```python
from build123d import *

# Parameters (mm, degrees)
F0_R     = 2.5
F1_DEPTH = 10
F2_W     = 10
F2_H     = 10
F3_DEPTH = 5
F5_DEPTH = 5


with BuildPart() as f1:
    # F0 (on Front) → F1 (new body)
    with BuildSketch(Plane.XZ):
        Circle(F0_R)
    extrude(amount=F1_DEPTH)

    # F2 (on face) → F3 (join)
    with BuildSketch(Plane.XZ.offset(10)):
        Rectangle(F2_W, F2_H)
    extrude(amount=F3_DEPTH)

    # F4 (on face) → F5 (cut, through all)
    with BuildSketch(Plane.XZ.offset(15)):
        Polygon((0, 5), (0, 0), (-5, 0), (-5, -5), (5, -5), (5, 0), (5, 5), align=None)
    extrude(amount=-F5_DEPTH, mode=Mode.SUBTRACT)


solid = f1.part
```
Verification items for the finished model (mm, model axes). A direction names the side the tool comes from. Coordinates: 2 decimals unless noted, no trailing zeros. Write each loop counter-clockwise with the first axis right and the second up, starting at its lowest first coordinate (ties: lowest second). Pieces come first, ordered by that corner, then holes. Notation, with made-up numbers: (-12, 36) - (45, 36) arc R29 ccw to (45, 58) - close; hole circle Ø11 at (88, 89). An arc over 180 degrees is marked (long way). Write item = value, one per line.
Q1. Go/stop test with flat-tipped pins: pin 1 Ø2.5 at (x, y) = (-3.5, -12) entering from -Z; pin 2 Ø1.5 at (x, y) = (-2, -8.5) entering from +Z; pin 3 Ø2.5 at (y, z) = (-12, 2.5) entering from +X. Record where each tip stops, or that it passes through.
Answer:
pin_1 = 0
pin_2 = 2.17
pin_3 = 0
Q2. Cross-section at D-D (z = 2.25). Enter the section's corners in (x, y).
Answer:
outline = (-5, -15) - (0, -15) - (0, -10) - (1.09, -10) - (1.09, 0) - (-1.09, 0) - (-1.09, -10) - (-5, -10) - close
Q3. Material ranges on L1, parallel to X at y = -14, z = 4.5; L2, parallel to Y at x = 0.75, z = -2; L3, parallel to Y at x = -3.5, z = 2, recorded low to high. Write a range as from..to.
Answer:
L1 = -5..0
L2 = -10..0
L3 = -15..-10
Q4. Cross-section at A-A (z = 0.25). Enter the section's corners in (x, y).
Answer:
outline = (-5, -15) - (0, -15) - (0, -10) - (2.49, -10) - (2.49, 0) - (-2.49, 0) - (-2.49, -10) - (-5, -10) - close
Q5. Mould release check, pull along Z, two halves, no side actions. Record for faces 1 (the face through (-5, -12, 2)), 2 (the face through (-2, -13, 0)), 3 (the face through (-3, -12, 5)), 4 (the face through (-0.54, -4.93, -2.44)): released by +Z, released by -Z, zero draft, split by the parting line, or undercut.
Answer:
face_1 = zero draft
face_2 = released by -Z
face_3 = released by +Z
face_4 = split by the parting line
Q6. Cross-section at B-B (y = -12.25). Enter the section's corners in (x, z).
Answer:
outline = (-5, 0) - (0, 0) - (0, 5) - (-5, 5) - close
Q7. Cross-section at C-C (x = 1.25). Enter the section's corners in (y, z), plus the area to 3 significant figures.
Answer:
outline = (-10, -2.17) - (0, -2.17) - (0, 2.17) - (-10, 2.17) - close
area = 43.3 mm²
Q8. Access from +Z, -Z, +X, -X, +Y, -Y to the whole of each face (thin tool, end or side, straight path). Record for faces 5 (the face through (0, -13, 3)), 6 (the face through (-3, -15, 3)), 7 (the face through (-3, -10, 3)).
Answer:
face_5 = +Z, -Z, +X, -Y
face_6 = +Z, -Z, +X, -X, -Y
face_7 = +Z, -X, +Y
